```python
from build123d import *

# Parameters (mm, degrees)
SKETCH2_W                   = 6.35
SKETCH2_H                   = 25.4
BOSS_EXTRUDE1_DEPTH         = 31.75
BOSS_EXTRUDE1_2_DEPTH       = 31.75
SKETCH2_3_W                 = 25.4
SKETCH2_3_H                 = 25.4
BOSS_EXTRUDE2_DEPTH         = 3.175
SKETCH3_R                   = 6.35
CUT_EXTRUDE1_DEPTH          = 56.72102386
SKETCH4_W                   = 25.4
SKETCH4_H                   = 6.35
BOSS_EXTRUDE3_DEPTH         = 12.7
SKETCH9_W                   = 25.4
SKETCH9_H                   = 6.35
BOSS_EXTRUDE5_DEPTH         = 12.7
F_1_4_20_TAPPED_HOLE3_D     = 5.1054
F_1_4_20_TAPPED_HOLE3_DEPTH = 19.05
F_1_4_20_TAPPED_HOLE3_TIP   = 1.533816902


with BuildPart() as part:
    # Sketch2 → Boss-Extrude1 (new body)
    with BuildSketch(Plane(origin=(0, 0, 0), x_dir=(1, 0, 0), z_dir=(0, 1, 0))):
        with Locations((3.175, 12.7)):
            Rectangle(SKETCH2_W, SKETCH2_H)
    extrude(amount=BOSS_EXTRUDE1_DEPTH)



with BuildPart() as body_2:
    # Sketch2 → Boss-Extrude1 2 (new body)
    with BuildSketch(Plane(origin=(0, 0, 0), x_dir=(1, 0, 0), z_dir=(0, 1, 0))):
        with Locations((34.925, 12.7)):
            Rectangle(SKETCH2_W, SKETCH2_H)
    extrude(amount=BOSS_EXTRUDE1_2_DEPTH)


with BuildPart() as part_1:
    add(part.part)

    add(body_2.part)  # Boss-Extrude2 merges body 2
    # Sketch2<3> → Boss-Extrude2 (add)
    with BuildSketch(Plane(origin=(0, 0, 0), x_dir=(1, 0, 0), z_dir=(0, 1, 0))):
        with Locations((19.05, 12.7)):
            Rectangle(SKETCH2_3_W, SKETCH2_3_H)
    extrude(amount=BOSS_EXTRUDE2_DEPTH)

    # Sketch3 → Cut-Extrude1 (cut, through all)
    with BuildSketch(Plane.ZY):
        with Locations((-12.7, 19.05)):
            Circle(SKETCH3_R)
    extrude(amount=-CUT_EXTRUDE1_DEPTH, mode=Mode.SUBTRACT)

    # Sketch4 → Boss-Extrude3 (add)
    with BuildSketch(Plane.ZY):
        with Locations((-12.7, 3.175)):
            Rectangle(SKETCH4_W, SKETCH4_H)
    extrude(amount=BOSS_EXTRUDE3_DEPTH)

    # Sketch9 → Boss-Extrude5 (add)
    with BuildSketch(Plane(origin=(38.1, 0, 0), x_dir=(0, 0, -1), z_dir=(1, 0, 0))):
        with Locations((12.7, 3.175)):
            Rectangle(SKETCH9_W, SKETCH9_H)
    extrude(amount=BOSS_EXTRUDE5_DEPTH)

    # 1/4-20 Tapped Hole3
    with Locations(Plane(origin=(-6.35, 6.35, -19.05), x_dir=(0, 0, 1), z_dir=(0, 1, 0))):
        with Locations((0, 0), (12.7, 0), (12.7, 50.8), (0, 50.8)):
            Hole(F_1_4_20_TAPPED_HOLE3_D / 2, depth=F_1_4_20_TAPPED_HOLE3_DEPTH)
            with Locations((0, 0, -(F_1_4_20_TAPPED_HOLE3_DEPTH + F_1_4_20_TAPPED_HOLE3_TIP / 2))):  # 118° drill point
                Cone(0, F_1_4_20_TAPPED_HOLE3_D / 2, F_1_4_20_TAPPED_HOLE3_TIP, mode=Mode.SUBTRACT)


solid = part_1.part
```
Geometry check sheet. Reference: the model listing, model coordinates, mm. A direction names the side the tool comes from. Give positions to 0.01 mm unless a question says otherwise; leave off trailing zeros. Write each loop counter-clockwise with the first axis right and the second up, starting at its lowest first coordinate (ties: lowest second). Pieces come first, ordered by that corner, then holes. Notation, with made-up numbers: (80.5, 89.5) -> (101.5, 89.5) arc R18 cw to (101.5, 96.5) -> close; hole circle Ø6 at (-40, 60.5). An arc over 180 degrees is marked (long way). Use one line per item in the form item = value.
Item 1: Access from +Z, -Z, +X, -X, +Y, -Y to the whole of each face (thin tool, end or side, straight path). Record for faces 4 (the flat face through (38.1, 13, -10)), 5 (the flat face through (19, 3.175, -13)), 6 (the flat face through (0, 13, -10)), 7 (the flat face through (19, 0, -13)).
Results list:
face_4 = +Z, -Z, +X, +Y
face_5 = +Z, -Z, +Y
face_6 = +Z, -Z, -X, +Y
face_7 = +Z, -Z, +X, -X, -Y
Item 2: Mould release check, pull along Y, two halves, no side actions. Record for faces 1 (the flat face through (44, 6.35, -13)), 2 (the flat face through (6.35, 11, -13)), 3 (the cylindrical face through (34.881, 24.404, -9.286)): released by +Y, released by -Y, zero draft, split by the parting line, or undercut.
Results list:
face_1 = released by +Y
face_2 = zero draft
face_3 = undercut
Item 3: Sectioned sample at D-D on y = 19.05. Enter the section's corners in (x, z).
Results list:
outline = (0, -25.4) -> (6.35, -25.4) -> (6.35, -19.05) -> (0, -19.05) -> close; (0, -6.35) -> (6.35, -6.35) -> (6.35, 0) -> (0, 0) -> close; (31.75, -25.4) -> (38.1, -25.4) -> (38.1, -19.05) -> (31.75, -19.05) -> close; (31.75, -6.35) -> (38.1, -6.35) -> (38.1, 0) -> (31.75, 0) -> close
Item 4: Scan lines: line 1 (X direction, y = 4, z = -6.35); line 2 (X direction, y = 2.25, z = -19.05); line 3 (Z direction, x = 44.45, y = 1.75). Record each from-to range of solid material in increasing order.
Results list:
line_1 = -12.7 to -8.9, -3.8 to 6.35, 31.75 to 41.9, 47 to 50.8
line_2 = -12.7 to -8.9, -3.8 to 41.9, 47 to 50.8
line_3 = -25.4 to -21.6, -16.5 to -8.9, -3.8 to 0
Item 5: Sectioned sample at B-B on y = 5. Enter the section's corners in (x, z), plus the area to 3 significant figures.
Results list:
outline = (-12.7, -25.4) -> (6.35, -25.4) -> (6.35, 0) -> (-12.7, 0) -> close; (31.75, -25.4) -> (50.8, -25.4) -> (50.8, 0) -> (31.75, 0) -> close; hole circle Ø5.11 at (-6.35, -19.05); hole circle Ø5.11 at (-6.35, -6.35); hole circle Ø5.11 at (44.45, -19.05); hole circle Ø5.11 at (44.45, -6.35)
area = 886 mm2
Item 6: Sectioned sample at C-C on x = -6.35. Enter the section's corners in (y, z), plus the area to 3 significant figures.
Results list:
outline = (0, -25.4) -> (6.35, -25.4) -> (6.35, -21.6) -> (0, -21.6) -> close; (0, -16.5) -> (6.35, -16.5) -> (6.35, -8.9) -> (0, -8.9) -> close; (0, -3.8) -> (6.35, -3.8) -> (6.35, 0) -> (0, 0) -> close
area = 96.5 mm2
Item 7: Depth check by flat-ended pin: pin 1 Ø4 at (x, z) = (44.5, -12) entering from +Y; pin 2 Ø12.5 at (x, z) = (13, -9.5) entering from +Y (3 decimals); pin 3 Ø4.5 at (x, z) = (-6.35, -19.05) entering from +Y; pin 4 Ø7.5 at (y, z) = (17.5, -7) entering from +X. Enter the tip coordinate at first touch or a pass-through.
Results list:
pin_1 = 6.35
pin_2 = 3.175
pin_3 = through
pin_4 = 38.1
Item 8: Sectioned sample at A-A on z = -12.7. Enter the section's corners in (x, y) (3 decimals).
Results list:
outline = (-12.7, 0) -> (50.8, 0) -> (50.8, 6.35) -> (38.1, 6.35) -> (38.1, 12.7) -> (31.75, 12.7) -> (31.75, 3.175) -> (6.35, 3.175) -> (6.35, 12.7) -> (0, 12.7) -> (0, 6.35) -> (-12.7, 6.35) -> close; (0, 25.4) -> (6.35, 25.4) -> (6.35, 31.75) -> (0, 31.75) -> close; (31.75, 25.4) -> (38.1, 25.4) -> (38.1, 31.75) -> (31.75, 31.75) -> close
